Check sheet for the modelled part. Datum: model origin and axes. Units: mm. Face numbers are marked on the shaded views. A direction names the side the tool comes from. Round coordinates to 2 decimals unless told otherwise and drop trailing zeros. Write each loop counter-clockwise with the first axis right and the second up, starting at its lowest first coordinate (ties: lowest second). Pieces come first, ordered by that corner, then holes.
Item 1: Cross-section at C-C on z = 28.5. Enter the section's corners in (x, y).
Item 2: Cross-section at B-B on x = 8. Enter the section's corners in (y, z), plus the area to 3 significant figures.
Item 3: Release check for a two-part mould opening along X. For the marked faces 3, 4, 5 and 6 record: +X half, -X half, draft (parallel to the pull), parting line (faces both ways), or undercut.
Item 4: Go/stop test with flat-tipped pins: pin 1 Ø6 at (y, z) = (-15, 25.5) entering from -X; pin 2 Ø5 at (y, z) = (-8.5, 13.5) entering from -X; pin 3 Ø8 at (y, z) = (-15, 28) entering from +X. Record where each tip stops, or that it passes through.
Item 5: Material ranges on line 1 (Z direction, x = 22, y = -5.75); line 2 (X direction, y = -2.25, z = 4); line 3 (X direction, y = -8.5, z = 2), recorded low to high.
Item 6: Tool access check on the marked faces 1 and 2. Record the directions out of +Z, -Z, +X, -X, +Y, -Y that give a thin tool (end or side, any length) a straight path to the whole face; none if there is none.
Item 7: Cross-section at A-A on y = -4. Enter the section's corners in (x, z), plus the area to 3 significant figures.
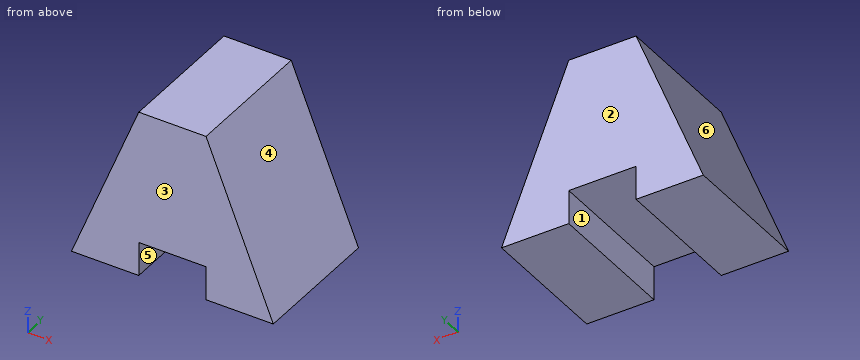
from build123d import *

# Parameters (mm, degrees)
F0_W     = 38.2099039853
F0_H     = 31.7133665085
F1_DEPTH = 25.4
F3_DEPTH = 25.401
F5_DEPTH = 25.401
F6_W     = 12.736634817
F6_H     = 6.4110578969
F7_DEPTH = 25.401


with BuildPart() as f1:
    # F0 (on Front) → F1 (new body)
    with BuildSketch(Plane.XZ):
        with Locations((19.1049519926, 15.8566832542)):
            Rectangle(F0_W, F0_H)
    extrude(amount=F1_DEPTH)

    # F2 (on face) → F3 (cut, through all)
    with BuildSketch(Plane.XZ.offset(25.4)):
        Polygon((0, 0), (12.7366343513, 31.7133665085), (0, 31.7133665085), align=None)
    extrude(amount=-F3_DEPTH, mode=Mode.SUBTRACT)

    # F4 (on face) → F5 (cut, through all)
    with BuildSketch(Plane.XZ.offset(25.4)):
        Polygon((38.2099039853, 31.7133665085), (25.4732691683, 31.7133665085), (38.2099039853, 0), align=None)
    extrude(amount=-F5_DEPTH, mode=Mode.SUBTRACT)

    # F6 (on face) → F7 (cut, through all)
    with BuildSketch(Plane.XZ.offset(25.4)):
        with Locations((19.1049517598, 3.2055289485)):
            Rectangle(F6_W, F6_H)
    extrude(amount=-F7_DEPTH, mode=Mode.SUBTRACT)


solid = f1.part
Response values:
1. outline: (11.45, -25.4) - (26.76, -25.4) - (26.76, 0) - (11.45, 0) - close
2. outline: (-25.4, 0) - (0, 0) - (0, 19.92) - (-25.4, 19.92) - close
2. area: 506 mm2
3. face 3: draft
3. face 4: +X half
3. face 5: undercut
3. face 6: -X half
4. pin 1: stops at x = 9.04
4. pin 2: stops at x = 4.42
4. pin 3: stops at x = 28.57
5. line 1: z = 6.41 to 31.71
5. line 2: x = 1.61 to 12.74, 25.47 to 36.6
5. line 3: x = 0.8 to 12.74, 25.47 to 37.41
6. face 1: -Z, +Y, -Y
6. face 2: +Z, -Z, +X, -X, +Y
7. outline: (0, 0) - (12.74, 0) - (12.74, 6.41) - (25.47, 6.41) - (25.47, 0) - (38.21, 0) - (25.47, 31.71) - (12.74, 31.71) - close
7. area: 726 mm2
